Verification items for the finished model (mm, model axes). A direction names the side the tool comes from. Round coordinates to 2 decimals unless told otherwise and drop trailing zeros. Order: outer loops, then holes, each group sorted by start corner. A loop starts at its lowest first (then second) coordinate and runs counter-clockwise, first axis right, second up. Notation, with made-up numbers: M 85,72 L 142,72 A30 ccw 142,95 Z; hole C 57,-40 d7. An arc over 180 degrees is marked long. Use one line per item in the form item = value. Start each with the question number.
Item 1: Cross-section at C-C on z = 26.5. Enter the section's corners in (x, y), then the cut area to 3 significant figures.
Item 2: Thickness scan on probe 1 along X at (y, z) = (-16.5, 7); probe 2 along Z at (x, y) = (33, 5.5); probe 3 along Z at (x, y) = (-8, 5.5). Record the ranges inside material, lowest first. Write a range as [from, to].
Item 3: Go/stop test with flat-tipped pins: pin 1 Ø7 at (x, y) = (26, -15.5) entering from +Z; pin 2 Ø2.5 at (y, z) = (17, 8) entering from +X; pin 3 Ø4.5 at (x, y) = (-26.96, 15.97) entering from -Z; pin 4 Ø5.5 at (y, z) = (-16, 9.5) entering from -X. Record where each tip stops, or that it passes through.
Item 4: Cross-section at A-A on z = 8.5. Count the separate pieces of the cut face and the enclosed holes in it, then the cut area to 3 significant figures.
Item 5: Release check for a two-part mould opening along Y. For faces 3 (the flat face through (29.26, 12.05, 9.04)), 4 (the flat face through (0, -9, 12)), 5 (the flat face through (-27.68, -12.12, 9.04)) record: +Y half, -Y half, draft (parallel to the pull), parting line (faces both ways), or undercut.
Item 6: Tool access check on faces 1 (the flat face through (-20.96, -16, 9)), 2 (the cylindrical face through (-23.076, -15.283, 2.958)). Record the directions out of +Z, -Z, +X, -X, +Y, -Y that give a thin tool (end or side, any length) a straight path to the whole face; none if there is none.
Item 7: Cross-section at B-B on z = 33. Enter the section's corners in (x, y).
from build123d import *

# Parameters (mm, degrees)
F0_R     = 2.5
F1_DEPTH = 12
F3_R     = 2.5
F4_DEPTH = 6
F8_R     = 2


# Not quite as in the source:
# - a fillet or chamfer that OpenCascade refuses, or shapes differently, is made with other operations: its cross-section is extruded or revolved along the edge and cut away or added


with BuildPart() as f1:
    # F0 (on Top) → F1 (new body)
    with BuildSketch(Plane.XY):
        with BuildLine():
            ThreePointArc((-31.3651592039, 24.7400687451), (-33.0304528025, 22.4689333996), (-34.5318159842, 20.0862527403))
            ThreePointArc((-34.5318159842, 20.0862527403), (0.3556410553, -40.0322385106), (34.289361103, 20.6296959515))
            ThreePointArc((34.289361103, 20.6296959515), (32.9313235996, 22.7293613836), (31.4447447441, 24.7400687451))
            add(Edge.make_bspline(
                [(31.4447447441, 24.7400687451), (22.988602022, 32.1085255021), (13.1297165658, 36.2919575894), (0.0397927701, 36.9132596428)],
                knots=[0, 0, 0, 0, 0.5, 0.5, 0.5, 0.5], degree=3))
            add(Edge.make_bspline(
                [(-31.3651592039, 24.7400687451), (-22.9090164817, 32.1085255021), (-13.0501310255, 36.2919575894), (0.0397927701, 36.9132596428)],
                knots=[0, 0, 0, 0, 0.5, 0.5, 0.5, 0.5], degree=3))
        make_face()
        with Locations((-25.4602072299, -16.0334855318)):
            Circle(F0_R, mode=Mode.SUBTRACT)
        with Locations((25.5397927701, -16.0334855318)):
            Circle(F0_R, mode=Mode.SUBTRACT)
        with Locations((-26.9602072299, 15.9665144682)):
            Circle(F0_R, mode=Mode.SUBTRACT)
        with Locations((27.0397927701, 15.9665144682)):
            Circle(F0_R, mode=Mode.SUBTRACT)
    extrude(amount=F1_DEPTH)

    # F3 (on face) → F4 (cut)
    with BuildSketch(Plane.XY.offset(12)):
        Polygon((-22.4602072299, 13.3684382568), (-22.4602072299, 18.5645906795), (-26.9602072299, 21.1626668909), (-31.4602072299, 18.5645906795), (-31.4602072299, 13.3684382568), (-26.9602072299, 10.7703620455), align=None)
        with Locations((-26.9602072299, 15.9665144682)):
            Circle(F3_R, mode=Mode.SUBTRACT)
        Polygon((22.5397927701, 18.5645906795), (22.5397927701, 13.3684382568), (27.0397927701, 10.7703620455), (31.5397927701, 13.3684382568), (31.5397927701, 18.5645906795), (27.0397927701, 21.1626668909), align=None)
        with Locations((27.0397927701, 15.9665144682)):
            Circle(F3_R, mode=Mode.SUBTRACT)
        Polygon((21.0397927701, -13.4354093205), (21.0397927701, -18.6315617432), (25.5397927701, -21.2296379545), (30.0397927701, -18.6315617432), (30.0397927701, -13.4354093205), (25.5397927701, -10.8373331091), align=None)
        with Locations((25.5397927701, -16.0334855318)):
            Circle(F3_R, mode=Mode.SUBTRACT)
        Polygon((-20.9602072299, -18.6315617432), (-20.9602072299, -13.4354093205), (-25.4602072299, -10.8373331091), (-29.9602072299, -13.4354093205), (-29.9602072299, -18.6315617432), (-25.4602072299, -21.2296379545), align=None)
        with Locations((-25.4602072299, -16.0334855318)):
            Circle(F3_R, mode=Mode.SUBTRACT)
    extrude(amount=-F4_DEPTH, mode=Mode.SUBTRACT)

    # F5 (on Front) → F6 (revolve)
    with BuildSketch(Plane.XZ):
        with BuildLine():
            Line((-8.284470181, 11.8907699668), (0, 11.8907699668))
            Line((0, 11.8907699668), (0, 48.1916638966))
            ThreePointArc((0, 48.1916638966), (-3.1039423325, 47.8080717015), (-6.0211163429, 46.6803763667))
            ThreePointArc((-6.0211163429, 46.6803763667), (-12.7413209188, 34.9713010104), (-5.1760724611, 23.7895922406))
            add(Edge.make_bspline(
                [(-8.284470181, 13.6864552548), (-7.2384952575, 14.7658121918), (-4.9346184441, 17.14342214), (-5.0921300249, 21.4398414936), (-5.1760724611, 23.7895922406)],
                knots=[0, 0, 0, 0, 0.4540341601, 1, 1, 1, 1], degree=3))
            Line((-8.284470181, 13.6864552548), (-8.284470181, 11.8907699668))
        make_face()
    revolve(axis=Axis((0, 0, 50.5361706018), (0, 0, 1)))

    # F7: fillet of radius 5 on 1 edges, made by hand

    # F7_s1 → F7_t2 (revolve, cut)
    with BuildSketch(Plane.XZ):
        with BuildLine():
            ThreePointArc((-8.284470181, 12), (-7.9344186734, 13.5789038819), (-7.0987068449, 14.9634829753))
            Line((-7.0987068449, 14.9634829753), (-7.1748362782, 15.0283236215))
            ThreePointArc((-7.1748362782, 15.0283236215), (-7.7543234481, 14.3838527889), (-8.3562826351, 13.7560467158))
            Line((-8.3562826351, 13.7560467158), (-8.384470181, 13.6864552548))
            ThreePointArc((-8.384470181, 13.6864552548), (-8.384470181, 12.8432276274), (-8.384314881, 12.0055709867))
            Line((-8.384314881, 12.0055709867), (-8.284470181, 12))
        make_face()
    revolve(axis=Axis((0, 0, 13.6864552548), (0, 0, 1)), mode=Mode.SUBTRACT)

    # F8
    f8_edges = [f1.edges().sort_by_distance(p)[0] for p in [
        (-2.459557, -39.955325, 12),
        (-2.459557, -39.955325, 0),
        (16.831403, 33.608309, 12),
        (-16.751817, 33.608309, 12),
        (-16.751817, 33.608309, 0),
        (16.831403, 33.608309, 0),
    ]]
    fillet(f8_edges, radius=F8_R)


solid = f1.part
Output values:
q1.outline = C 0,0 d18.18
q1.area = 260 mm2
q2.probe_1 = [-36.41, -29.96], [-20.96, 21.04], [30.04, 36.49]
q2.probe_2 = [0, 12]
q2.probe_3 = [0, 12], [27.18, 43.71]
q3.pin_1 = 6
q3.pin_2 = 36.79
q3.pin_3 = through
q3.pin_4 = -37.71
q4.separate_pieces = 1
q4.enclosed_holes = 4
q4.area = 4,600 mm2
q5.face_3 = undercut
q5.face_4 = draft
q5.face_5 = undercut
q6.face_1 = +Z
q6.face_2 = +Z, -Z
q7.outline = C 0,0 d25.03
